Work out the finished part from the listing and answer in its coordinate system (mm). A direction names the side the tool comes from. Give positions to 0.01 mm unless a question says otherwise; leave off trailing zeros. Order: outer loops, then holes, each group sorted by start corner. A loop starts at its lowest first (then second) coordinate and runs counter-clockwise, first axis right, second up. Notation, with made-up numbers: (54.25, 54) - (59.25, 54) arc R24 ccw to (59.25, 88) - close; hole circle Ø2 at (28.25, 27). An arc over 180 degrees is marked (long way). Put each result on its own line as item: value.
```python
from build123d import *

# Parameters (mm, degrees)
F0_W     = 102.6246032535
F0_H     = 89.4768349826
F1_DEPTH = 55.626
F3_DEPTH = 141.224
F4_DEPTH = 156.718
F5_R     = 11.6889879412
F6_DEPTH = 134.874
F7_R     = 11.1336119635
F8_DEPTH = 268.478


with BuildPart() as f1:
    # F0 (on Top) → F1 (new body, symmetric)
    with BuildSketch(Plane.XY):
        with Locations((-9.000580439, 1.2215245515)):
            Rectangle(F0_W, F0_H)
    extrude(amount=F1_DEPTH, both=True)

    # F2 (on face) → F3 (join)
    with BuildSketch(Plane.XY.offset(55.626)):
        with BuildLine():
            ThreePointArc((-30.4661283079, 45.9599420428), (-6.615057122, 22.1088708569), (17.2360140639, 45.9599420428))
            Line((17.2360140639, 45.9599420428), (8.524204708, 45.9599420428))
            ThreePointArc((8.524204708, 45.9599420428), (-6.615057122, 30.8206802129), (-21.7543189519, 45.9599420428))
            Line((-21.7543189519, 45.9599420428), (-30.4661283079, 45.9599420428))
        make_face()
    extrude(amount=-F3_DEPTH)

    # F4 (cut): a face of the model
    f4_faces = [f1.faces().sort_by_distance(p)[0] for p in [
        (-6.615057122, 39.5346397628, -55.626),
    ]]
    extrude(f4_faces, amount=-F4_DEPTH, mode=Mode.SUBTRACT)

    # F5 (on face) → F6 (cut, symmetric)
    with BuildSketch(Plane(origin=(0, 45.9599420428, 0), x_dir=(-1, 0, 0), z_dir=(0, 1, 0))):
        with Locations((-27.0718317479, 0)):
            Circle(F5_R)
    extrude(amount=F6_DEPTH, both=True, mode=Mode.SUBTRACT)

    # F7 (on face) → F8 (cut)
    with BuildSketch(Plane(origin=(0, 45.9599420428, 0), x_dir=(-1, 0, 0), z_dir=(0, 1, 0))):
        with Locations((40.8077836037, 0)):
            Circle(F7_R)
    extrude(amount=-F8_DEPTH, mode=Mode.SUBTRACT)


solid = f1.part
```
(1) Determine the mould class of faces 3 (the face through (-6.948, 30.824, -15.975)), 4 (the face through (-51.43, 1.85, 3.34)), 5 (the face through (36.35, 1.85, -7.11)), 6 (the face through (-10, 2, 55.626)) for opening direction Z: pulls with the +Z half, pulls with the -Z half, needs draft (parallel to the pull), parting line crosses it, or undercut.
Geometry check:
face 3: needs draft
face 4: undercut
face 5: undercut
face 6: pulls with the +Z half
(2) Given pin 1 (1 mm diameter, centred on x = -46.5, y = -23.5, fed in from -Z), flat-ended and moving along its own axis, determine where the tip first touches the part or whether it passes through.
Geometry check:
pin 1: stops at z = -55.63
(3) Section C-C, the plane z = -52 is taken. Write down the section's boundary in (x, y).
Geometry check:
outline: (-60.31, -43.52) - (42.31, -43.52) - (42.31, 45.96) - (8.52, 45.96) arc R15.14 cw to (-21.75, 45.96) - (-60.31, 45.96) - close
(4) Section D-D, the plane x = -47 is taken. Write down the section's boundary in (y, z).
Geometry check:
outline: (-43.52, -55.63) - (45.96, -55.63) - (45.96, -9.25) - (-43.52, -9.25) - close; (-43.52, 9.25) - (45.96, 9.25) - (45.96, 55.63) - (-43.52, 55.63) - close
(5) Straight lines are drawn through the part: line 1 (Z direction, x = 27, y = 32.5); line 2 (Z direction, x = 30.5, y = 37); line 3 (X direction, y = 22.5, z = -9). For each, find the intervals that lie inside material, in ascending order.
Geometry check:
line 1: z = -55.63 to -11.69, 11.69 to 55.63
line 2: z = -55.63 to -11.17, 11.17 to 55.63
line 3: x = -60.31 to -47.36, -34.25 to 19.61, 34.53 to 42.31
(6) Section A-A, the plane z = 0 is taken. Write down the section's boundary in (x, y), then the cut area to 3 significant figures.
Geometry check:
outline: (-60.31, -43.52) - (-51.94, -43.52) - (-51.94, 45.96) - (-60.31, 45.96) - close; (-29.67, -43.52) - (15.38, -43.52) - (15.38, 45.96) - (8.52, 45.96) arc R15.14 cw to (-21.75, 45.96) - (-29.67, 45.96) - close; (38.76, -43.52) - (42.31, -43.52) - (42.31, 45.96) - (38.76, 45.96) - close
area: 4,740 mm²
(7) A tool of negligible diameter and unlimited length cuts with its end or side. For faces 1 (the face through (-7.14, 22.115, -70.402)), 2 (the face through (-10, -43.517, 1)), from which of +Z, -Z, +X, -X, +Y, -Y can it reach the whole face along a straight path? Write none if from no direction.
Geometry check:
face 1: -Z, -Y
face 2: +Z, -Z, +X, -X, -Y
(8) Section B-B, the plane y = 14 is taken. Write down the section's boundary in (x, z).
Geometry check:
outline: (-60.31, -55.63) - (42.31, -55.63) - (42.31, 55.63) - (-60.31, 55.63) - close; hole circle Ø22.27 at (-40.81, 0); hole circle Ø23.38 at (27.07, 0)
